For this review, take the finished solid that the model builds, in its own axes (mm). Give positions to 0.01 mm unless a question says otherwise; leave off trailing zeros. Write each loop counter-clockwise with the first axis right and the second up, starting at its lowest first coordinate (ties: lowest second). Pieces come first, ordered by that corner, then holes.
1) We need section A-A on y = 3.9. Give the boundary of the cut face in (x, z), and give its area (3 significant figures).
2) We need section B-B on y = 0.45. Give the number of separate pieces and of enclosed holes in the cut face, and give its area (3 significant figures).
3) Wall thickness on line 1 along X through (y, z) = (5.15, -1); line 2 along Y through (x, z) = (-3.25, 1.25); line 3 along Z through (x, y) = (2.25, 1.95): over which ranges is each line inside the solid? List them lowest first.
4) Draft analysis for pull direction X (two halves, no side actions). For faces 1 (the face through (-0.874, 2.712, 3.935)), 2 (the face through (-0.841, 0.37, 3.788)), state which applies: pulls with the +X half, pulls with the -X half, needs draft (parallel to the pull), parting line crosses it, or undercut.
5) For P1, Ø1.5, axis at x = -3, z = 2.5, coming from the +Y side; P2, Ø1, axis at y = 4.5, z = -1, coming from the -X side; P3, Ø2, axis at x = 2, z = 2, coming from the +Y side, all flat-tipped, find the tip position at first contact; note any pin that passes through.
from build123d import *

# Parameters (mm, degrees)
SKETCH1_R                = 4.03065
SKETCH1_R_2              = 3.88065
BOSS_EXTRUDE1_DEPTH      = 5.5
SKETCH3_R                = 0.197408615
BOSS_EXTRUDE2_DEPTH      = 0.28159739
BOSS_EXTRUDE2_DEPTH_BACK = 5.5


with BuildPart() as part:
    # Sketch1 → Boss-Extrude1 (new body)
    with BuildSketch(Plane(origin=(0, 0, 0), x_dir=(1, 0, 0), z_dir=(0, 1, 0))):
        Circle(SKETCH1_R)
        Circle(SKETCH1_R_2, mode=Mode.SUBTRACT)
    extrude(amount=BOSS_EXTRUDE1_DEPTH)

    # Sketch2 → Revolve1 (revolve)
    with BuildSketch(Plane.XY):
        with BuildLine():
            Line((0.197408615, 0), (0.197408615, 5.781917471))
            ThreePointArc((0.197408615, 5.781917471), (2.106547816, 5.506953748), (3.88065, 4.75))
            Line((3.88065, 4.75), (3.88065, 0.75))
            ThreePointArc((3.88065, 0.75), (2.068627273, 0.229644733), (0.197408615, 0))
        make_face()
    revolve(axis=Axis((0, 5.5, 0), (0, -1, 0)))

    # Sketch3 → Boss-Extrude2 (add, two sides)
    with BuildSketch(Plane(origin=(0, 5.5, 0), x_dir=(1, 0, 0), z_dir=(0, 1, 0))) as boss_extrude2_sk:
        Circle(SKETCH3_R)
    extrude(amount=BOSS_EXTRUDE2_DEPTH)
    extrude(boss_extrude2_sk.sketch, amount=-BOSS_EXTRUDE2_DEPTH_BACK)


solid = part.part
Results list:
1. outline: circle Ø8.06 at (0, 0)
1. area: 51.0 mm2
2. separate pieces: 2
2. enclosed holes: 1
2. area: 31.4 mm2
3. line 1: x = -3.9 to -3.75, -2.94 to 2.94, 3.75 to 3.9
3. line 2: y = 0.61 to 4.97
3. line 3: z = -3.34 to 3.34
4. face 1: parting line crosses it
4. face 2: undercut
5. P1: stops at y = 5.5
5. P2: stops at x = -4
5. P3: stops at y = 5.58
